Input: dimensioned drawing with shaded views. Units: mm. Origin: part minimum x, y, z. A direction names the side the tool comes from. Give positions to 0.01 mm unless a question says otherwise; leave off trailing zeros. Loops run counter-clockwise (first coordinate to the right, second up) from the corner with the lowest first, then second, coordinate; pieces in that order, holes last.
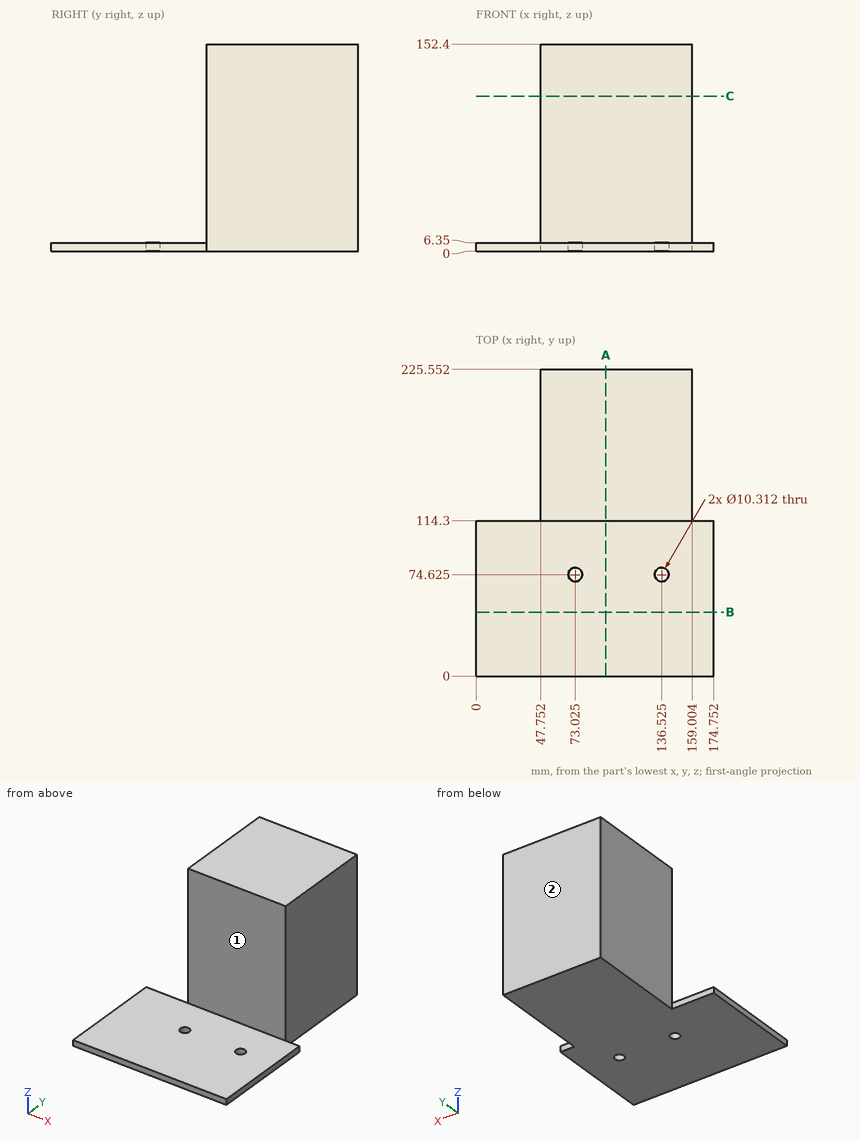
(1) Ray query, line 1 along Z through (x, y) = (29, 95); line 2 along Y through (x, z) = (154.5, 112); line 3 along X through (y, z) = (165, 29). Return the intervals inside material, ascending.
A:
line 1: z = 0 to 6.35
line 2: y = 114.3 to 225.55
line 3: x = 47.75 to 159
(2) Section C-C, the plane z = 114. Return the cut outline in (x, y).
A:
outline: (47.75, 114.3) - (159, 114.3) - (159, 225.55) - (47.75, 225.55) - close
(3) Section B-B, the plane y = 47. Return the cut outline in (x, z), then the cut area to 3 significant figures.
A:
outline: (0, 0) - (174.75, 0) - (174.75, 6.35) - (0, 6.35) - close
area: 1,110 mm2
(4) First-contact query: pin 1 (4 mm diameter, centred on x = 156.5, z = 46.5, fed in from -Y); pin 2 (16.5 mm diameter, centred on x = 73.03, y = 74.63, fed in from +Z); pin 3 (5 mm diameter, centred on x = 170, z = 2, fed in from +Y). Flat tips, straight axial feed; report the tip coordinate or a pass-through.
A:
pin 1: stops at y = 114.3
pin 2: stops at z = 6.35
pin 3: stops at y = 114.3
(5) Reachability of the marked faces 1 and 2 from +Z, -Z, +X, -X, +Y, -Y: full face, straight path, thin tool, end or side. Return the list, or none.
A:
face 1: +Z, +X, -X, -Y
face 2: +Z, -Z, +X, -X, +Y
(6) Section A-A, the plane x = 95.5. Return the cut outline in (y, z), then the cut area to 3 significant figures.
A:
outline: (0, 0) - (225.55, 0) - (225.55, 152.4) - (114.3, 152.4) - (114.3, 6.35) - (0, 6.35) - close
area: 17,700 mm2
